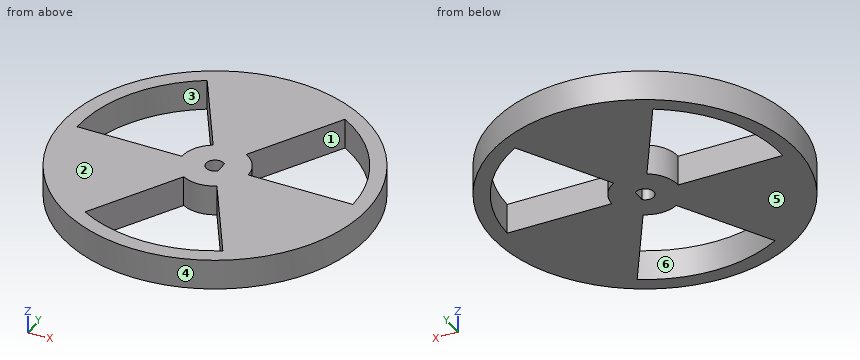
```python
from build123d import *

# Parameters (mm, degrees)
ESQUISSE1_R        = 60
BOSS_EXTRU_1_DEPTH = 12
CUT_EXTRUDE1_DEPTH = 12


with BuildPart() as part:
    # Esquisse1 → Boss.-Extru.1 (new body)
    with BuildSketch(Plane.XY):
        Circle(ESQUISSE1_R)
        with BuildLine():
            ThreePointArc((13, 0), (11.258330249, 6.5), (6.5, 11.258330249))
            Line((6.5, 11.258330249), (27, 46.765371804))
            ThreePointArc((27, 46.765371804), (46.765371804, 27), (54, 0))
            Line((54, 0), (13, 0))
        make_face(mode=Mode.SUBTRACT)
        with BuildLine():
            Line((-27, 46.765371804), (-6.5, 11.258330249))
            ThreePointArc((-6.5, 11.258330249), (-11.258330249, 6.5), (-13, 0))
            Line((-13, 0), (-54, 0))
            ThreePointArc((-54, 0), (-46.765371804, 27), (-27, 46.765371804))
        make_face(mode=Mode.SUBTRACT)
        with BuildLine():
            Line((-27, -46.765371804), (-6.5, -11.258330249))
            ThreePointArc((-6.5, -11.258330249), (0, -13), (6.5, -11.258330249))
            Line((6.5, -11.258330249), (27, -46.765371804))
            ThreePointArc((27, -46.765371804), (0, -54), (-27, -46.765371804))
        make_face(mode=Mode.SUBTRACT)
    extrude(amount=BOSS_EXTRU_1_DEPTH)

    # Sketch1 → Cut-Extrude1 (cut)
    with BuildSketch(Plane.XY.offset(12)):
        with BuildLine():
            Line((2.449489743, 2.5), (2.449489743, -2.5))
            ThreePointArc((2.449489743, -2.5), (-3.5, 0), (2.449489743, 2.5))
        make_face()
    extrude(amount=-CUT_EXTRUDE1_DEPTH, mode=Mode.SUBTRACT)


solid = part.part
```
CAD build for the part. Positions are in the model's coordinates, mm. Face numbers are marked on the shaded views. A direction names the side the tool comes from. Coordinates: 2 decimals unless noted, no trailing zeros. Order: outer loops, then holes, each group sorted by start corner. A loop starts at its lowest first (then second) coordinate and runs counter-clockwise, first axis right, second up. Notation, with made-up numbers: (3.5, 68.25) - (43.5, 68.25) arc R19 cw to (43.5, 84.25) - close; hole circle Ø4 at (7.5, 27.25). An arc over 180 degrees is marked (long way). Use a Markdown table: item, result. Add a question column.
(1) Saw through at B-B (y = -21.5). Give the cut face in (x, z).
(2) Saw through at A-A (z = 8.25). Give the cut face in (x, y), then the cut area to 3 significant figures.
(3) Saw through at D-D (x = -39.5). Give the cut face in (y, z).
(4) Flat gauge pins, fed straight in: pin 1 (4 mm diameter, centred on x = 22, z = 3.5, fed in from -Y); pin 2 (1 mm diameter, centred on x = -36.5, z = 1.5, fed in from +Y); pin 3 (3.5 mm diameter, centred on x = -24.5, z = 8.5, fed in from +Y); pin 4 (1.5 mm diameter, centred on x = 43.5, y = 29.5, fed in from +Z). Where does each tip first touch, or does it go through?
(5) Pull direction Y, two halves, no side cores. Call the marked faces 1, 2, 3 and 4: +Y half, -Y half, draft (parallel to the pull), parting line (faces both ways), or undercut.
(6) Drill centre lines: line 1 along Y through (x, z) = (0, 5.75); line 2 along X through (y, z) = (21.5, 10); line 3 along X through (y, z) = (44, 11). Where is each one in solid material? Low to high. Write a range as [from, to].
(7) Saw through at C-C (x = 0). Give the cut face in (y, z).
(8) Which spindle directions (+Z, -Z, +X, -X, +Y, -Y) get a long thin tool onto all of the face, cutting with end or side? Do the marked faces 5 and 6. Say none if no direction does.
Solved:
| question | item | result |
|---|---|---|
| 1 | outline | (-56.02, 0) - (-12.41, 0) - (-12.41, 12) - (-56.02, 12) - close; (12.41, 0) - (56.02, 0) - (56.02, 12) - (12.41, 12) - close |
| 2 | outline | circle Ø120 at (0, 0); hole (-54, 0) - (-13, 0) arc R13 cw to (-6.5, 11.26) - (-27, 46.77) arc R54 ccw to start; hole (-27, -46.77) arc R54 ccw to (27, -46.77) - (6.5, -11.26) arc R13 cw to (-6.5, -11.26) - close; hole (2.45, -2.5) - (2.45, 2.5) arc R3.5 ccw (long way) to start; hole (6.5, 11.26) arc R13 cw to (13, 0) - (54, 0) arc R54 ccw to (27, 46.77) - close |
| 2 | area | 6,960 mm² |
| 3 | outline | (-45.16, 0) - (0, 0) - (0, 12) - (-45.16, 12) - close; (36.82, 0) - (45.16, 0) - (45.16, 12) - (36.82, 12) - close |
| 4 | pin 1 | stops at y = -56.57 |
| 4 | pin 2 | stops at y = 48 |
| 4 | pin 3 | stops at y = 55.52 |
| 4 | pin 4 | passes through |
| 5 | face 1 | undercut |
| 5 | face 2 | draft |
| 5 | face 3 | undercut |
| 5 | face 4 | parting line |
| 6 | line 1 | y = [-60, -54], [-13, -3.5], [3.5, 60] |
| 6 | line 2 | x = [-56.02, -49.54], [-12.41, 12.41], [49.54, 56.02] |
| 6 | line 3 | x = [-40.79, -31.3], [-25.4, 25.4], [31.3, 40.79] |
| 7 | outline | (-60, 0) - (-54, 0) - (-54, 12) - (-60, 12) - close; (-13, 0) - (-3.5, 0) - (-3.5, 12) - (-13, 12) - close; (3.5, 0) - (60, 0) - (60, 12) - (3.5, 12) - close |
| 8 | face 5 | -Z, +X, -X, +Y, -Y |
| 8 | face 6 | +Z, -Z |
